Build history of the part. All positions in model axes, mm. A direction names the side the tool comes from. Round coordinates to 2 decimals unless told otherwise and drop trailing zeros. Loops run counter-clockwise (first coordinate to the right, second up) from the corner with the lowest first, then second, coordinate; pieces in that order, holes last. Notation, with made-up numbers: (-8, 40) - (27, 40) arc R24 cw to (27, 59) - close; hole circle Ø7 at (87.5, 77.25). An arc over 180 degrees is marked (long way). Answer as CSV lines item,"result". Start each with the question number.
```python
from build123d import *

# Parameters (mm, degrees)
F0_W      = 25.4
F0_H      = 25.3999925918
F1_DEPTH  = 17.78
F2_DEPTH  = 25.4
F3_W      = 17.78
F3_H      = 25.4
F4_DEPTH  = 15.24
F6_DEPTH  = 25.4
F7_W      = 25.4
F7_H      = 25.4
F8_DEPTH  = 17.78
F9_W      = 25.4
F9_H      = 17.78
F10_DEPTH = 50.8
F11_W     = 25.4
F11_H     = 25.4
F12_DEPTH = 25.4


with BuildPart() as f1:
    # F0 (on Right) → F1 (new body)
    with BuildSketch(Plane.YZ):
        with Locations((39.7640056908, 21.4484632015)):
            Rectangle(F0_W, F0_H)
    extrude(amount=F1_DEPTH)

    # F2 (add): a face of the model
    f2_faces = [f1.faces().sort_by_distance(p)[0] for p in [
        (8.89, 27.0640056908, 21.4484632015),
    ]]
    extrude(f2_faces, amount=F2_DEPTH)

    # F3 (on face) → F4 (join)
    with BuildSketch(Plane(origin=(0, 0, 8.7484669056), x_dir=(1, 0, 0), z_dir=(0, 0, -1))):
        with Locations((8.89, -14.3640056908)):
            Rectangle(F3_W, F3_H)
    extrude(amount=F4_DEPTH)

    # F5 (on face) → F6 (join)
    with BuildSketch(Plane(origin=(0, 0, 0), x_dir=(0, -1, 0), z_dir=(-1, 0, 0))):
        Polygon((-27.0640056908, 34.1484594974), (-27.0640056908, 8.7484669056), (-27.0640056908, -6.4915330944), (-1.6640056908, -6.4915330944), (-1.6640056908, 34.1484594974), align=None)
    extrude(amount=F6_DEPTH)

    # F7 (on face) → F8 (join)
    with BuildSketch(Plane.XY.offset(34.1484594974)):
        with Locations((-12.7, 14.3640056908)):
            Rectangle(F7_W, F7_H)
    extrude(amount=F8_DEPTH)

    # F9 (on face) → F10 (join)
    with BuildSketch(Plane(origin=(-25.4, 0, 0), x_dir=(0, -1, 0), z_dir=(-1, 0, 0))):
        with Locations((-14.3640056908, 43.0384594974)):
            Rectangle(F9_W, F9_H)
    extrude(amount=F10_DEPTH)

    # F11 (on face) → F12 (join)
    with BuildSketch(Plane(origin=(0, 0, 34.1484594974), x_dir=(1, 0, 0), z_dir=(0, 0, -1))):
        with Locations((-63.5, -14.3640056908)):
            Rectangle(F11_W, F11_H)
    extrude(amount=F12_DEPTH)


solid = f1.part
```
Q1. Wall check: probe 1 along X at (y, z) = (19, 14.5); probe 2 along X at (y, z) = (37.5, 23); probe 3 along X at (y, z) = (10.5, 1.5). Give the ranges that are in metal, low to high. Write a range as [from, to].
Q2. Band-saw the part on C-C, the plane y = 10. List the corners of the cut face in (x, z).
Q3. Tool access for faces 1 (the flat face through (-25.4, 14, 14)), 2 (the flat face through (0, 14, 43)), 3 (the flat face through (9, 40, 8.748)), 4 (the flat face through (0, 40, 22)): list every direction of +Z, -Z, +X, -X, +Y, -Y with a clear straight run to the whole face (end or side of a thin tool).
Q4. Band-saw the part on D-D, the plane z = 47. List the corners of the cut face in (x, y).
Q5. Two-plate mould, pull along X, no slides. Class faces 5 (the flat face through (-64, 14, 8.748)), 6 (the flat face through (-50.8, 15, 22)), 7 (the flat face through (17.78, 27, 19)): released by +X, released by -X, zero draft, split by the parting line, or undercut.
Q6. Pin check, flat tips, straight feed: pin 1 Ø20.5 at (y, z) = (39.5, 20) entering from -X; pin 2 Ø12.5 at (x, y) = (-67, 16) entering from -Z; pin 3 Ø12 at (x, z) = (-53.5, 42.5) entering from +Y; pin 4 Ø1 at (x, z) = (-49, 24) entering from +Y. Stop position of each tip, or through.
Q7. Band-saw the part on A-A, the plane z = 29. List the corners of the cut face in (x, y).
Q8. Band-saw the part on B-B, the plane x = 4.5. List the corners of the cut face in (y, z).
Reported:
1,probe 1,"x = [-76.2, -50.8], [-25.4, 17.78]"
1,probe 2,"x = [0, 17.78]"
1,probe 3,"x = [-25.4, 17.78]"
2,outline,"(-76.2, 8.75) - (-50.8, 8.75) - (-50.8, 34.15) - (-25.4, 34.15) - (-25.4, -6.49) - (17.78, -6.49) - (17.78, 34.15) - (0, 34.15) - (0, 51.93) - (-76.2, 51.93) - close"
3,face 1,"-Z, +Y, -Y"
3,face 2,"+Z, +X, +Y, -Y"
3,face 3,"-Z, +X, -X, +Y"
3,face 4,"+Z, -Z, -X, +Y"
4,outline,"(-76.2, 1.66) - (0, 1.66) - (0, 27.06) - (-76.2, 27.06) - close"
5,face 5,"zero draft"
5,face 6,"undercut"
5,face 7,"released by +X"
6,pin 1,"stops at x = 0"
6,pin 2,"stops at z = 8.75"
6,pin 3,"stops at y = 27.06"
6,pin 4,"passes through"
7,outline,"(-76.2, 1.66) - (-50.8, 1.66) - (-50.8, 27.06) - (-76.2, 27.06) - close; (-25.4, 1.66) - (17.78, 1.66) - (17.78, 52.46) - (0, 52.46) - (0, 27.06) - (-25.4, 27.06) - close"
8,outline,"(1.66, -6.49) - (27.06, -6.49) - (27.06, 8.75) - (52.46, 8.75) - (52.46, 34.15) - (1.66, 34.15) - close"
